Work out the finished part from the listing and answer in its coordinate system (mm). A direction names the side the tool comes from. Coordinates: 2 decimals unless noted, no trailing zeros. Loops run counter-clockwise (first coordinate to the right, second up) from the corner with the lowest first, then second, coordinate; pieces in that order, holes last. Notation, with made-up numbers: (78.5, 80.25) - (119.5, 80.25) arc R14 ccw to (119.5, 107.25) - close; hole circle Ø5 at (71.5, -35). An arc over 180 degrees is marked (long way). Write each question's results on one line, items separated by ' | '. Start each with the question number.
1. A cutting plane is placed at A-A on z = 13.4. Determine the outline of the cut face in (x, y).
2. Each of these flat-tipped pins is pushed along its axis until it touches: P1, Ø2.5, axis at x = -1, z = -6.5, coming from the -Y side; P2, Ø4, axis at x = -1.5, y = 20, coming from the -Z side; P3, Ø2.5, axis at x = -0.5, z = 14.5, coming from the -Y side; P4, Ø3, axis at x = -0.5, z = -0.5, coming from the +Y side. Where does it stop, or does it pass through?
3. Which of the six approach directions +Z, -Z, +X, -X, +Y, -Y give full straight-line access (tool end or side, diameter ignored) to faces 1 (the flat face through (0, 19, 11.4)), 2 (the flat face through (0, 15, 15)), 3 (the cylindrical face through (-0.716, 23.972, -11.353))?
4. Find the intervals of material crossed by line 1 along Z through (x, y) = (0, 16.1); line 2 along X through (y, z) = (16.1, 13.4); line 3 along Y through (x, z) = (4.75, 10.5), in increasing order. Write a range as [from, to].
5. A cutting plane is placed at B-B on x = 2. Determine the outline of the cut face in (y, z).
6. Determine the mould class of faces 4 (the flat face through (0, 17, -15)), 5 (the cylindrical face through (-0.54, 29.14, -3.26)), 6 (the cylindrical face through (0.45, 27.31, -7.13)) for opening direction Y: released by +Y, released by -Y, zero draft, split by the parting line, or undercut.
7. A cutting plane is placed at D-D on x = -3.75. Determine the outline of the cut face in (y, z).
8. A cutting plane is placed at C-C on y = 21. Determine the outline of the cut face in (x, z), then the cut area to 3 significant figures.
from build123d import *

# Parameters (mm, degrees)
SKETCH2_W           = 12.2
SKETCH2_H           = 22.8
BOSS_EXTRUDE1_DEPTH = 22
SKETCH3_W           = 12.2
SKETCH3_H           = 4.6
SKETCH3_R           = 1
BOSS_EXTRUDE2_DEPTH = 2
SKETCH4_R           = 5.5
BOSS_EXTRUDE3_DEPTH = 4
SKETCH5_R           = 2.5
BOSS_EXTRUDE4_DEPTH = 4.2
SKETCH6_W           = 1
SKETCH6_H           = 1.6


with BuildPart() as part:
    # Sketch2 → Boss-Extrude1 (new body)
    with BuildSketch(Plane(origin=(0, 0, 0), x_dir=(1, 0, 0), z_dir=(0, 1, 0))):
        Rectangle(SKETCH2_W, SKETCH2_H)
    extrude(amount=BOSS_EXTRUDE1_DEPTH)

    # Sketch3 → Boss-Extrude2 (add)
    with BuildSketch(Plane(origin=(0, 15, 0), x_dir=(1, 0, 0), z_dir=(0, 1, 0))):
        with Locations((0, 13.7)):
            Rectangle(SKETCH3_W, SKETCH3_H)
        with Locations((0, 13.4)):
            Circle(SKETCH3_R, mode=Mode.SUBTRACT)
        with Locations((0, -13.7)):
            Rectangle(SKETCH3_W, SKETCH3_H)
        with Locations((0, -13.4)):
            Circle(SKETCH3_R, mode=Mode.SUBTRACT)
    extrude(amount=BOSS_EXTRUDE2_DEPTH)

    # Sketch4 → Boss-Extrude3 (add)
    with BuildSketch(Plane(origin=(0, 22, 0), x_dir=(1, 0, 0), z_dir=(0, 1, 0))):
        with Locations((0, 5.9)):
            Circle(SKETCH4_R)
    extrude(amount=BOSS_EXTRUDE3_DEPTH)

    # Sketch5 → Boss-Extrude4 (add)
    with BuildSketch(Plane(origin=(0, 26, 0), x_dir=(1, 0, 0), z_dir=(0, 1, 0))):
        with Locations((0, 5.7)):
            Circle(SKETCH5_R)
    extrude(amount=BOSS_EXTRUDE4_DEPTH)

    # Sketch6 → Cut-Revolve1 (revolve, cut)
    with BuildSketch(Plane(origin=(0, 0, 0), x_dir=(0, 0, -1), z_dir=(1, 0, 0))):
        with Locations((7.7, 27.3)):
            Rectangle(SKETCH6_W, SKETCH6_H)
    revolve(axis=Axis((0, 30.2, -5.7), (0, -1, 0)), mode=Mode.SUBTRACT)


solid = part.part
Values:
1) outline: (-6.1, 15) - (-1, 15) - (-1, 17) - (-6.1, 17) - close; (1, 15) - (6.1, 15) - (6.1, 17) - (1, 17) - close
2) P1: y = 0 | P2: z = -11.4 | P3: y = 15 | P4: y = 26
3) face 1: +Z, +X, -X, +Y | face 2: +Z, +X, -X, -Y | face 3: +Y
4) line 1: [-16, -14.4], [-12.4, 12.4], [14.4, 16] | line 2: [-6.1, -1], [1, 6.1] | line 3: [0, 22]
5) outline: (0, -11.4) - (15, -11.4) - (15, -16) - (17, -16) - (17, -11.4) - (22, -11.4) - (22, -11.02) - (26, -11.02) - (26, -7.2) - (26.5, -7.2) - (26.5, -4.2) - (26, -4.2) - (26, -0.78) - (22, -0.78) - (22, 11.4) - (17, 11.4) - (17, 16) - (15, 16) - (15, 11.4) - (0, 11.4) - close; (28.1, -7.2) - (30.2, -7.2) - (30.2, -4.2) - (28.1, -4.2) - close
6) face 4: released by +Y | face 5: zero draft | face 6: undercut
7) outline: (0, -11.4) - (15, -11.4) - (15, -16) - (17, -16) - (17, -11.4) - (22, -11.4) - (22, -9.92) - (26, -9.92) - (26, -1.88) - (22, -1.88) - (22, 11.4) - (17, 11.4) - (17, 16) - (15, 16) - (15, 11.4) - (0, 11.4) - close
8) outline: (-6.1, -11.4) - (6.1, -11.4) - (6.1, 11.4) - (-6.1, 11.4) - close | area: 278 mm^2
